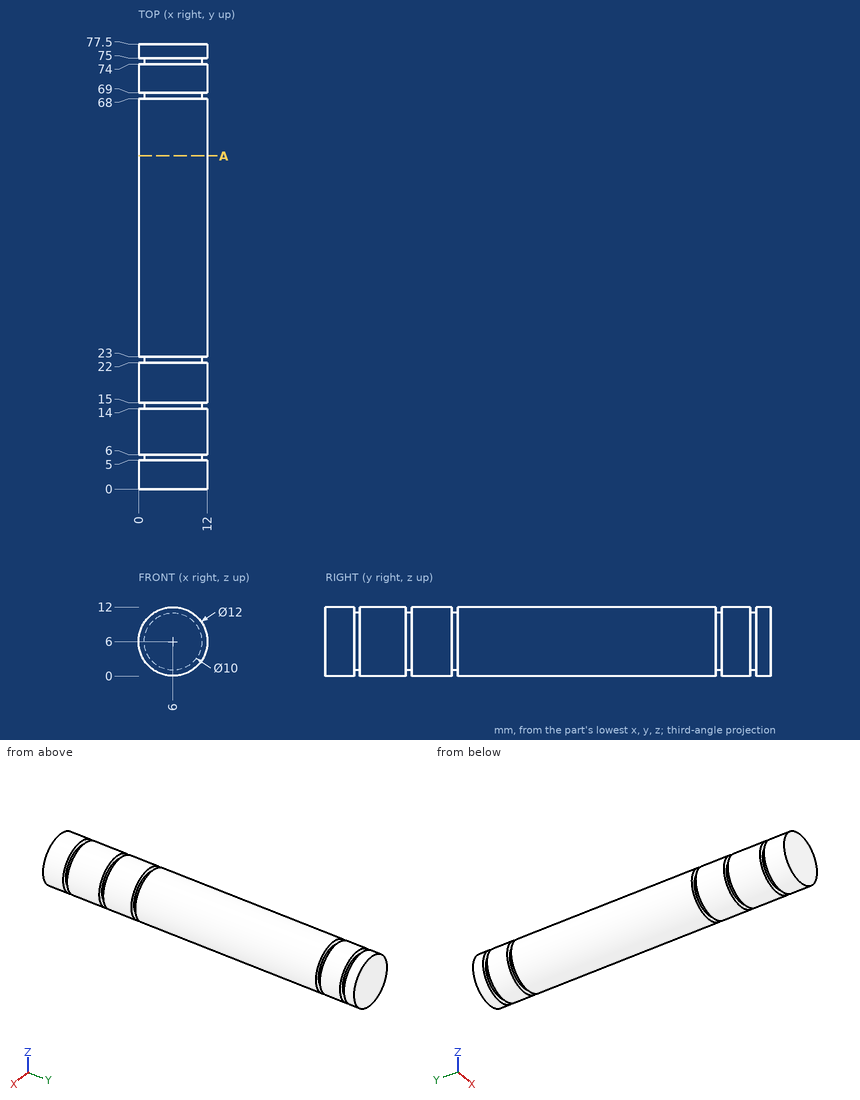
For this review, use the dimensioned drawing (mm, ordinates from the lowest corner) and the shaded views. Give positions to 0.01 mm unless a question says otherwise; leave off trailing zeros. Order: outer loops, then holes, each group sorted by start corner. A loop starts at its lowest first (then second) coordinate and runs counter-clockwise, first axis right, second up.
1) Take a section at A-A (y = 58). Give the boundary of the cut face in (x, z), then the cut area to 3 significant figures.
2) Wall thickness on line 1 (Y direction, x = 3.75, z = 0.75); line 2 (Z direction, x = 6.25, y = 63); line 3 (X direction, y = 66, z = 7): over which ranges is each line inside the solid? List them lowest first.
3) Insertion check: pin 1 (1.5 mm diameter, centred on y = 16.5, z = 7.5, fed in from +X); pin 2 (2 mm diameter, centred on y = 29.5, z = 8.5, fed in from -X); pin 3 (2 mm diameter, centred on x = 1, y = 41.5, fed in from +Z). Each pin has a flat end and moves straight along its axis. Give the tip position at first contact, or say it passes through.
Derived:
1. outline: circle Ø12 at (6, 6)
1. area: 113 mm2
2. line 1: y = 0 to 5, 6 to 14, 15 to 22, 23 to 68, 69 to 74, 75 to 77.5
2. line 2: z = 0.01 to 11.99
2. line 3: x = 0.08 to 11.92
3. pin 1: stops at x = 11.95
3. pin 2: stops at x = 0.19
3. pin 3: stops at z = 10.47
